from build123d import *

# Parameters (mm, degrees)
SKETCH1_R           = 3.515
BOSS_EXTRUDE1_DEPTH = 50
SKETCH2_R           = 2.5
BOSS_EXTRUDE2_DEPTH = 10
SKETCH3_R           = 2.5
BOSS_EXTRUDE5_DEPTH = 60


with BuildPart() as part:
    # Sketch1 → Boss-Extrude1 (new body)
    with BuildSketch(Plane(origin=(0, 0, 0), x_dir=(1, 0, 0), z_dir=(0, 1, 0))):
        Circle(SKETCH1_R)
    extrude(amount=BOSS_EXTRUDE1_DEPTH)

    # Sketch2 → Boss-Extrude2 (add)
    with BuildSketch(Plane(origin=(0, 0, 0), x_dir=(1, 0, 0), z_dir=(0, 1, 0))):
        Circle(SKETCH2_R)
    extrude(amount=-BOSS_EXTRUDE2_DEPTH)

    # Sketch3 → Boss-Extrude5 (add)
    with BuildSketch(Plane(origin=(0, 0, 0), x_dir=(1, 0, 0), z_dir=(0, 1, 0))):
        Circle(SKETCH3_R)
    extrude(amount=BOSS_EXTRUDE5_DEPTH)


solid = part.part
Verification items for the finished model (mm, model axes). A direction names the side the tool comes from. Coordinates: 2 decimals unless noted, no trailing zeros. Order: outer loops, then holes, each group sorted by start corner. A loop starts at its lowest first (then second) coordinate and runs counter-clockwise, first axis right, second up. Notation, with made-up numbers: M -18,-1.75 L 3,-1.75 A14 cw 3,25.25 Z; hole C -13.5,77.25 d4. An arc over 180 degrees is marked long. Write each question's results on one line, items separated by ' | '.
1) Gauge pin test, flat ends, axial feed: pin 1 Ø2 at (y, z) = (31, -2.5) entering from -X; pin 2 Ø1 at (y, z) = (33, -1) entering from -X. Record the tip position at first contact, or that the pin passes through.
Solved:
pin 1: stops at x = -3.18 | pin 2: stops at x = -3.48
2) Section check A-A on x = 0. Record the cut outline in (y, z) (3 decimals).
Solved:
outline: M -10,-2.5 L 0,-2.5 L 0,-3.515 L 50,-3.515 L 50,-2.5 L 60,-2.5 L 60,2.5 L 50,2.5 L 50,3.515 L 0,3.515 L 0,2.5 L -10,2.5 Z
3) Access from +Z, -Z, +X, -X, +Y, -Y to the whole of each face (thin tool, end or side, straight path). Record for faces 1 (the face through (0, 60, 0)), 2 (the face through (-0.54, 54.93, 2.44)), 3 (the face through (2, 0, 2)).
Solved:
face 1: +Z, -Z, +X, -X, +Y | face 2: +Y | face 3: -Y
4) Scan lines: line 1 along Z through (x, y) = (-0.25, -1.5); line 2 along Y through (x, z) = (0.25, 2.75); line 3 along X through (y, z) = (46, -0.25). Record each from-to range of solid material in increasing order. Write a range as [from, to].
Solved:
line 1: z = [-2.49, 2.49] | line 2: y = [0, 50] | line 3: x = [-3.51, 3.51]
5) Section check B-B on y = 2.5. Record the cut outline in (x, z) (3 decimals), plus the area to 3 significant figures.
Solved:
outline: C 0,0 d7.03 | area: 38.8 mm²
